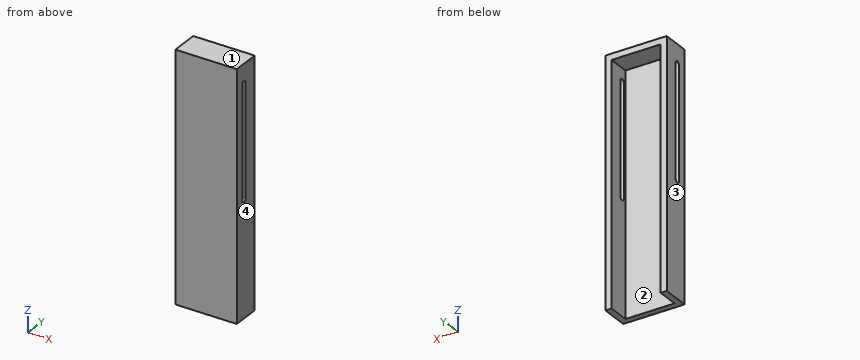
from build123d import *

# Parameters (mm, degrees)
SKETCH1_W           = 50
SKETCH1_H           = 200
BOSS_EXTRUDE1_DEPTH = 20
SKETCH2_W           = 40
SKETCH2_H           = 35
CUT_EXTRUDE1_DEPTH  = 190
SKETCH3_W           = 40
SKETCH3_H           = 17.5
CUT_EXTRUDE2_DEPTH  = 5
SKETCH4_W           = 50
SKETCH4_H           = 2.5
BOSS_EXTRUDE2_DEPTH = 200
CUT_EXTRUDE4_DEPTH  = 200
BOSS_EXTRUDE3_DEPTH = 50
SKETCH15_W          = 40
SKETCH15_H          = 4.25
CUT_EXTRUDE5_DEPTH  = 104
CUT_EXTRUDE6_DEPTH  = 104
BOSS_EXTRUDE4_DEPTH = 50
SKETCH19_W          = 40
SKETCH19_H          = 4.25
CUT_EXTRUDE7_DEPTH  = 50


with BuildPart() as part:
    # Sketch1 → Boss-Extrude1 (new body)
    with BuildSketch(Plane(origin=(0, 0, 0), x_dir=(1, 0, 0), z_dir=(0, 1, 0))):
        Rectangle(SKETCH1_W, SKETCH1_H)
    extrude(amount=BOSS_EXTRUDE1_DEPTH)

    # Sketch2 → Cut-Extrude1 (cut)
    with BuildSketch(Plane(origin=(0, 0, -100), x_dir=(-1, 0, 0), z_dir=(0, 0, -1))):
        with Locations((0, 20)):
            Rectangle(SKETCH2_W, SKETCH2_H)
    extrude(amount=-CUT_EXTRUDE1_DEPTH, mode=Mode.SUBTRACT)

    # Sketch3 → Cut-Extrude2 (cut)
    with BuildSketch(Plane(origin=(0, 0, 90), x_dir=(-1, 0, 0), z_dir=(0, 0, -1))):
        with Locations((0, 11.25)):
            Rectangle(SKETCH3_W, SKETCH3_H)
    extrude(amount=-CUT_EXTRUDE2_DEPTH, mode=Mode.SUBTRACT)

    # Sketch4 → Boss-Extrude2 (add)
    with BuildSketch(Plane(origin=(0, 0, -100), x_dir=(-1, 0, 0), z_dir=(0, 0, -1))):
        with Locations((0, -1.25)):
            Rectangle(SKETCH4_W, SKETCH4_H)
    extrude(amount=-BOSS_EXTRUDE2_DEPTH)

    # Sketch6 → Cut-Extrude4 (cut)
    with BuildSketch(Plane.ZY.offset(25)):
        with BuildLine():
            Line((90.75, 4.5), (-95.75, 4.5))
            ThreePointArc((-95.75, 4.5), (-97.875, 6.625), (-95.75, 8.75))
            Line((-95.75, 8.75), (90.75, 8.75))
            ThreePointArc((90.75, 8.75), (92.875, 6.625), (90.75, 4.5))
        make_face()
    extrude(amount=-CUT_EXTRUDE4_DEPTH, mode=Mode.SUBTRACT)

    # Sketch14 → Boss-Extrude3 (add)
    with BuildSketch(Plane.ZY.offset(25)):
        with BuildLine():
            Line((-0.375, 4.5), (-100, 4.5))
            Line((-100, 4.5), (-100, 8.75))
            Line((-100, 8.75), (-0.375, 8.75))
            ThreePointArc((-0.375, 8.75), (-2.5, 6.625), (-0.375, 4.5))
        make_face()
    extrude(amount=-BOSS_EXTRUDE3_DEPTH)

    # Sketch15 → Cut-Extrude5 (cut)
    with BuildSketch(Plane(origin=(0, 0, -100), x_dir=(-1, 0, 0), z_dir=(0, 0, -1))):
        with Locations((0, 6.625)):
            Rectangle(SKETCH15_W, SKETCH15_H)
    extrude(amount=-CUT_EXTRUDE5_DEPTH, mode=Mode.SUBTRACT)

    # Sketch17 → Cut-Extrude6 (cut)
    with BuildSketch(Plane.ZY.offset(25)):
        with BuildLine():
            Line((-0.375, 8.75), (-0.375, 4.5))
            Line((-0.375, 4.5), (-6.75, 4.5))
            ThreePointArc((-6.75, 4.5), (-8.875, 6.625), (-6.75, 8.75))
            Line((-6.75, 8.75), (-0.375, 8.75))
        make_face()
    extrude(amount=-CUT_EXTRUDE6_DEPTH, mode=Mode.SUBTRACT)

    # Sketch18 → Boss-Extrude4 (add)
    with BuildSketch(Plane.ZY.offset(25)):
        with BuildLine():
            Line((84.375, 4.5), (90.75, 4.5))
            ThreePointArc((90.75, 4.5), (92.875, 6.625), (90.75, 8.75))
            Line((90.75, 8.75), (84.375, 8.75))
            ThreePointArc((84.375, 8.75), (86.5, 6.625), (84.375, 4.5))
        make_face()
    extrude(amount=-BOSS_EXTRUDE4_DEPTH)

    # Sketch19 → Cut-Extrude7 (cut)
    with BuildSketch(Plane(origin=(0, 0, 95), x_dir=(-1, 0, 0), z_dir=(0, 0, -1))):
        with Locations((0, 6.625)):
            Rectangle(SKETCH19_W, SKETCH19_H)
    extrude(amount=CUT_EXTRUDE7_DEPTH, mode=Mode.SUBTRACT)


solid = part.part
Here's how the part is built. I have some questions about the finished solid (model axes, mm). Face numbers are marked on the shaded views. Round coordinates to 2 decimals unless told otherwise and drop trailing zeros. Order: outer loops, then holes, each group sorted by start corner. A loop starts at its lowest first (then second) coordinate and runs counter-clockwise, first axis right, second up. Notation, with made-up numbers: M -7.5,-31.75 L 22.5,-31.75 A22 ccw 22.5,-8.75 Z; hole C 27,-10 d4. An arc over 180 degrees is marked long. One line per question, with ' | ' between items.
1) Imagine slicing it at C-C, the plane z = -38. Write out the boundary of the cut face in (x, y).
Checked values:
outline: M -25,-2.5 L 25,-2.5 L 25,20 L 20,20 L 20,2.5 L -20,2.5 L -20,20 L -25,20 Z
2) I need wall thicknesses on line 1 (X direction, y = 10, z = -55); line 2 (Z direction, x = 8.5, y = 16); line 3 (Y direction, x = 8, z = 30). Which ranges of each line are inside material? Lowest first, please.
Checked values:
line 1: x = -25 to -20, 20 to 25 | line 2: z = 95 to 100 | line 3: y = -2.5 to 2.5
3) Imagine slicing it at B-B, the plane y = 17. Write out the boundary of the cut face in (x, z).
Checked values:
outline: M -25,-100 L -20,-100 L -20,95 L 20,95 L 20,-100 L 25,-100 L 25,100 L -25,100 Z
4) I'm going to push flat-ended pins straight in: pin 1 Ø8 at (x, z) = (1, 69) entering from +Y; pin 2 Ø1 at (x, y) = (-4, 8.5) entering from -Z. Where does each tip first touch, or does it pass through?
Checked values:
pin 1: stops at y = 2.5 | pin 2: stops at z = 95
5) Imagine slicing it at A-A, the plane z = 20. Write out the boundary of the cut face in (x, y), plus the area to 4 significant figures.
Checked values:
outline: M -25,-2.5 L 25,-2.5 L 25,4.5 L 20,4.5 L 20,2.5 L -20,2.5 L -20,4.5 L -25,4.5 Z; M -25,8.75 L -20,8.75 L -20,20 L -25,20 Z; M 20,8.75 L 25,8.75 L 25,20 L 20,20 Z | area: 382.5 mm²
6) Imagine slicing it at D-D, the plane x = -8. Write out the boundary of the cut face in (y, z), plus the area to 3 significant figures.
Checked values:
outline: M -2.5,-100 L 2.5,-100 L 2.5,95 L 20,95 L 20,100 L -2.5,100 Z | area: 1,090 mm²
7) We'd pull the mould along X, two halves only. Please class the marked faces 1, 2, 3 and 4: released by +X, released by -X, zero draft, split by the parting line, or undercut.
Checked values:
face 1: zero draft | face 2: undercut | face 3: released by -X | face 4: released by +X
